For this review, take the finished solid that the model builds, in its own axes (mm). Give positions to 0.01 mm unless a question says otherwise; leave off trailing zeros. Order: outer loops, then holes, each group sorted by start corner. A loop starts at its lowest first (then second) coordinate and runs counter-clockwise, first axis right, second up.
Item 1: Consider section C-C (z = 467). Give the boundary of the cut face in (x, y), plus the area to 3 significant figures.
Item 2: For probe 1 along Y at (x, z) = (2.95, 380); probe 2 along Z at (x, y) = (4.25, -609); probe 3 along Z at (x, y) = (3.8, -658), list the stretches that pass through material, from the lowest coordinate up.
Item 3: For P1, Ø2, axis at x = 2, y = -801, coming from the -Z side; P2, Ø1.4, axis at x = 1.5, z = 563, coming from the -Y side; P3, Ø2, axis at x = 3, y = -801, coming from the +Z side, all flat-tipped, find the tip position at first contact; note any pin that passes through.
Item 4: Consider section A-A (x = 3.85). Give the number of separate pieces and of enclosed holes in the cut face, plus the area to 3 significant figures.
Item 5: Consider section B-B (y = -582.5). Give the boundary of the cut face in (x, z), plus the area to 3 significant figures.
```python
from build123d import *

# Parameters (mm, degrees)
F0_W     = 5
F0_H     = 4.5
F1_DEPTH = 4.8


# Not quite as in the source:
# - a feature names something its author has since deleted; it is built from what else it names


with BuildPart() as f1:
    # F0 (on Right) → F1 (new body)
    with BuildSketch(Plane.YZ):
        Polygon((-531.3379881175, 344.0831357297), (-531.3379881175, 329.0831357297), (-526.3379881175, 329.0831357297), (-526.3379881175, 584.6633606824), (-531.3379881175, 584.6633606824), (-531.3379881175, 569.6633606824), (-531.3379881175, 559.6633606824), (-531.3379881175, 354.0831357297), align=None)
        Polygon((-611.2895517261, 584.6633606824), (-637.7260949769, 424.1829931527), (-639.3722244459, 414.1903303575), (-634.2269114077, 414.6633606824), (-621.0372525622, 494.7298534546), (-620.224537093, 499.6633606824), (-619.4118216237, 504.5968679101), (-606.2221627782, 584.6633606824), align=None)
        Polygon((-803.6983604223, 344.0831357297), (-803.6983604223, 329.0831357297), (-672.5181742699, 329.0831357297), (-672.5181742699, 324.5831357297), (-662.5181742699, 324.5831357297), (-662.5181742699, 329.0831357297), (-531.3379881175, 329.0831357297), (-531.3379881175, 344.0831357297), (-535.8379881175, 344.0831357297), (-535.8379881175, 354.0831357297), (-531.3379881175, 354.0831357297), (-531.3379881175, 559.6633606824), (-535.8379881175, 559.6633606824), (-535.8379881175, 569.6633606824), (-531.3379881175, 569.6633606824), (-531.3379881175, 584.6633606824), (-563.7800754478, 584.6633606824), (-568.7800754478, 584.6633606824), (-573.7800754478, 584.6633606824), (-606.2221627782, 584.6633606824), (-619.4118216237, 504.5968679101), (-614.9716651188, 503.8654239878), (-615.784380588, 498.93191676), (-616.5970960573, 493.9984095323), (-621.0372525622, 494.7298534546), (-634.2269114077, 414.6633606824), (-639.3722244459, 414.1903303575), (-649.1639211663, 413.2901383873), (-659.1219276721, 412.3746568573), (-778.9973858727, 401.3540004817), (-788.9553923784, 400.4385189517), (-803.6983604223, 399.0831357297), (-803.6983604223, 384.0831357297), (-799.1983604223, 384.0831357297), (-799.1983604223, 374.0831357297), (-803.6983604223, 374.0831357297), (-803.6983604223, 354.0831357297), (-799.1983604223, 354.0831357297), (-799.1983604223, 344.0831357297), align=None)
        Polygon((-808.6983604223, 329.0831357297), (-803.6983604223, 329.0831357297), (-803.6983604223, 344.0831357297), (-803.6983604223, 354.0831357297), (-803.6983604223, 374.0831357297), (-803.6983604223, 384.0831357297), (-803.6983604223, 399.0831357297), (-808.6983604223, 399.0831357297), (-808.6983604223, 374.0831357297), (-808.6983604223, 354.0831357297), align=None)
        Polygon((-808.6983604223, 403.4437065252), (-808.6983604223, 399.0831357297), (-803.6983604223, 399.0831357297), (-788.9553923784, 400.4385189517), (-789.3673590669, 404.9196218792), (-779.4093525612, 405.8351034093), (-778.9973858727, 401.3540004817), (-659.1219276721, 412.3746568573), (-659.5338943606, 416.8557597849), (-649.5758878549, 417.7712413149), (-649.1639211663, 413.2901383873), (-639.3722244459, 414.1903303575), (-637.7260949769, 424.1829931527), (-650.0610930658, 423.0489847629), (-808.6983604223, 408.4647918168), align=None)
        with Locations((-566.2800754478, 586.9133606824)):
            Rectangle(F0_W, F0_H)
        with Locations((-571.2800754478, 586.9133606824)):
            Rectangle(F0_W, F0_H)
    extrude(amount=F1_DEPTH)


solid = f1.part
```
Resolved:
1. outline: (0, -630.67) - (4.8, -630.67) - (4.8, -526.34) - (0, -526.34) - close
1. area: 501 mm2
2. probe 1: y = -808.7 to -803.7, -799.2 to -526.34
2. probe 2: z = 329.08 to 584.66
2. probe 3: z = 329.08 to 412.48, 417 to 422.32
3. P1: stops at z = 329.08
3. P2: stops at y = -614.97
3. P3: stops at z = 409.26
4. separate pieces: 1
4. enclosed holes: 7
4. area: 41,000 mm2
5. outline: (0, 329.08) - (4.8, 329.08) - (4.8, 584.66) - (0, 584.66) - close
5. area: 1,230 mm2
